```python
from build123d import *

# Parameters (mm, degrees)
ESBO_O1_W                = 200
ESBO_O1_H                = 150
RESSALTO_EXTRUS_O1_DEPTH = 20
ESBO_O4_W                = 185
ESBO_O4_H                = 135
CORTE_EXTRUS_O2_DEPTH    = 17
ESBO_O3_W                = 190
ESBO_O3_H                = 140
CORTE_EXTRUS_O3_DEPTH    = 3
ESBO_O6_R                = 10
CORTE_EXTRUS_O4_DEPTH    = 18
FILETE4_R                = 5
FILETE5_R                = 5
FILETE6_R                = 5
FILETE7_R                = 5
ESBO_O7_W                = 156.679491924
ESBO_O7_H                = 8
CORTE_EXTRUS_O5_DEPTH    = 300
ESBO_O8_W                = 8
ESBO_O8_H                = 106.679491924
CORTE_EXTRUS_O6_DEPTH    = 300
ESBO_O15_W               = 1.5
ESBO_O15_H               = 100
ESBO_O15_W_2             = 150
ESBO_O15_H_2             = 2
ESBO_O15_W_3             = 3.5
CORTE_EXTRUS_O7_DEPTH    = 2.5


with BuildPart() as part:
    # Esboço1 → Ressalto-extrusão1 (new body)
    with BuildSketch(Plane.XY):
        Rectangle(ESBO_O1_W, ESBO_O1_H)
    extrude(amount=RESSALTO_EXTRUS_O1_DEPTH)

    # Esboço4 → Corte-extrusão2 (cut)
    with BuildSketch(Plane.XY.offset(20)):
        Rectangle(ESBO_O4_W, ESBO_O4_H)
    extrude(amount=-CORTE_EXTRUS_O2_DEPTH, mode=Mode.SUBTRACT)

    # Esboço3 → Corte-extrusão3 (cut)
    with BuildSketch(Plane.XY.offset(20)):
        Rectangle(ESBO_O3_W, ESBO_O3_H)
    extrude(amount=-CORTE_EXTRUS_O3_DEPTH, mode=Mode.SUBTRACT)

    # Esboço6 → Corte-extrusão4 (cut)
    with BuildSketch(Plane.XY.offset(20)):
        with Locations((-95, 70)):
            Circle(ESBO_O6_R)
        with Locations((95, 70)):
            Circle(ESBO_O6_R)
        with Locations((-95, -70)):
            Circle(ESBO_O6_R)
        with Locations((95, -70)):
            Circle(ESBO_O6_R)
    extrude(amount=-CORTE_EXTRUS_O4_DEPTH, mode=Mode.SUBTRACT)

    # Filete4
    filete4_edges = [part.edges().sort_by_distance(p)[0] for p in [
        (-100, 75, 1),
    ]]
    fillet(filete4_edges, radius=FILETE4_R)

    # Filete5
    filete5_edges = [part.edges().sort_by_distance(p)[0] for p in [
        (100, 75, 1),
    ]]
    fillet(filete5_edges, radius=FILETE5_R)

    # Filete6
    filete6_edges = [part.edges().sort_by_distance(p)[0] for p in [
        (100, -75, 1),
    ]]
    fillet(filete6_edges, radius=FILETE6_R)

    # Filete7
    filete7_edges = [part.edges().sort_by_distance(p)[0] for p in [
        (-100, -75, 1),
    ]]
    fillet(filete7_edges, radius=FILETE7_R)

    # Esboço7 → Corte-extrusão5 (cut)
    with BuildSketch(Plane.XZ.offset(75)):
        with Locations((0, 10)):
            Rectangle(ESBO_O7_W, ESBO_O7_H)
    extrude(amount=-CORTE_EXTRUS_O5_DEPTH, mode=Mode.SUBTRACT)

    # Esboço8 → Corte-extrusão6 (cut)
    with BuildSketch(Plane.ZY.offset(100)):
        with Locations((10, 0)):
            Rectangle(ESBO_O8_W, ESBO_O8_H)
    extrude(amount=-CORTE_EXTRUS_O6_DEPTH, mode=Mode.SUBTRACT)

    # Esboço15 → Corte-extrusão7 (cut)
    with BuildSketch(Plane.XY.offset(20)):
        with Locations((-97.25, 0)):
            Rectangle(ESBO_O15_W, ESBO_O15_H)
        with Locations((0, 72.5)):
            Rectangle(ESBO_O15_W_2, ESBO_O15_H_2)
        with Locations((0, -72.5)):
            Rectangle(ESBO_O15_W_2, ESBO_O15_H_2)
        with Locations((96.25, 0)):
            Rectangle(ESBO_O15_W_3, ESBO_O15_H)
    extrude(amount=-CORTE_EXTRUS_O7_DEPTH, mode=Mode.SUBTRACT)


solid = part.part
```
Work out the finished part from the listing and answer in its coordinate system (mm). A direction names the side the tool comes from. Coordinates: 2 decimals unless noted, no trailing zeros. Loops run counter-clockwise (first coordinate to the right, second up) from the corner with the lowest first, then second, coordinate; pieces in that order, holes last. Notation, with made-up numbers: (1.25, -40) - (5.25, -40) arc R4 ccw to (5.25, -36) - close; hole circle Ø9 at (7.25, 89). An arc over 180 degrees is marked (long way). Use a Markdown table: item, result.
Item 1: Consider probe 1 along Y at (x, z) = (48.5, 18.5); probe 2 along X at (y, z) = (-35, 3.5); probe 3 along Y at (x, z) = (82.5, 16). Determine where each line is inside the solid, lowest interval first. Write a range as from..to.
Evaluation:
| item | result |
|---|---|
| probe 1 | y = -75..-73.5, -71.5..-70, 70..71.5, 73.5..75 |
| probe 2 | x = -100..-92.5, 92.5..100 |
| probe 3 | y = -75..-67.5, 67.5..75 |
Item 2: Find section B-B, the plane z = 8.5. State how many separate pieces and enclosed holes the cut face has, and give its area (3 significant figures).
Evaluation:
| item | result |
|---|---|
| separate pieces | 8 |
| enclosed holes | 0 |
| area | 419 mm2 |
Item 3: For faces 1 (the flat face through (-1, 71, 14)), 2 (the flat face through (-96, -1, 14)), 3 (the flat face through (92.5, -1, 15)), 4 (the flat face through (-1, 1, 3)), determine the directions among +Z, -Z, +X, -X, +Y, -Y from which every point of the face is accessible in a straight line to the end or side of a thin tool.
Evaluation:
| item | result |
|---|---|
| face 1 | +Y, -Y |
| face 2 | +X, -X |
| face 3 | +Z, +Y, -Y |
| face 4 | +Z |
Item 4: Find section C-C, the plane x = -16. Determine the outline of the cut face in (y, z), and give its area (3 significant figures).
Evaluation:
| item | result |
|---|---|
| outline | (-75, 0) - (75, 0) - (75, 6) - (67.5, 6) - (67.5, 3) - (-67.5, 3) - (-67.5, 6) - (-75, 6) - close; (-75, 14) - (-67.5, 14) - (-67.5, 17) - (-70, 17) - (-70, 20) - (-71.5, 20) - (-71.5, 17.5) - (-73.5, 17.5) - (-73.5, 20) - (-75, 20) - close; (67.5, 14) - (75, 14) - (75, 20) - (73.5, 20) - (73.5, 17.5) - (71.5, 17.5) - (71.5, 20) - (70, 20) - (70, 17) - (67.5, 17) - close |
| area | 560 mm2 |
Item 5: Given pin 1 Ø4 at (y, z) = (-4.5, 13.5) entering from -X; pin 2 Ø1.5 at (x, z) = (68.5, 7) entering from -Y; pin 3 Ø2 at (x, z) = (97, 18.5) entering from +Y; pin 4 Ø4.5 at (x, y) = (-89, -69) entering from +Z, each flat-ended and moving along its own axis, determine where each tip first touches the part or whether it passes through.
Evaluation:
| item | result |
|---|---|
| pin 1 | stops at x = -100 |
| pin 2 | passes through |
| pin 3 | stops at y = 60.46 |
| pin 4 | stops at z = 2 |
Item 6: Find section A-A, the plane y = 11. Determine the outline of the cut face in (x, z).
Evaluation:
| item | result |
|---|---|
| outline | (-100, 0) - (100, 0) - (100, 6) - (92.5, 6) - (92.5, 3) - (-92.5, 3) - (-92.5, 6) - (-100, 6) - close; (-100, 14) - (-92.5, 14) - (-92.5, 17) - (-95, 17) - (-95, 20) - (-96.5, 20) - (-96.5, 17.5) - (-98, 17.5) - (-98, 20) - (-100, 20) - close; (92.5, 14) - (100, 14) - (100, 20) - (98, 20) - (98, 17.5) - (95, 17.5) - (95, 17) - (92.5, 17) - close |
Item 7: The mould has two halves that part along X. Classify faces 5 (the flat face through (-96, -53.34, 10)), 6 (the cylindrical face through (-99, 73, 1)), 7 (the flat face through (-92.5, -1, 15)): +X half, -X half, draft (parallel to the pull), parting line (faces both ways), or undercut.
Evaluation:
| item | result |
|---|---|
| face 5 | draft |
| face 6 | -X half |
| face 7 | undercut |
